Here's how the part is built. I have some questions about the finished solid (model axes, mm). A direction names the side the tool comes from. Give positions to 0.01 mm unless a question says otherwise; leave off trailing zeros. Loops run counter-clockwise (first coordinate to the right, second up) from the corner with the lowest first, then second, coordinate; pieces in that order, holes last. Notation, with made-up numbers: (62, 57.25) - (70, 57.25) arc R27 cw to (70, 75.25) - close; hole circle Ø5 at (56.25, -5). An arc over 180 degrees is marked (long way). Use one line per item in the form item = value.
from build123d import *

# Parameters (mm, degrees)
SKETCH1_R                = 24.193
SKETCH1_R_2              = 20.193
BOSS_EXTRUDE1_DEPTH      = 24
CUT_EXTRUDE1_DEPTH       = 24
BOSS_EXTRUDE2_DEPTH      = 24
SKETCH4_R                = 4
CUT_EXTRUDE2_DEPTH       = 24
SKETCH6_R                = 4
BOSS_EXTRUDE3_DEPTH      = 9.2
BOSS_EXTRUDE3_DEPTH_BACK = 11
SKETCH6_5_R              = 4
CUT_EXTRUDE4_DEPTH       = 4.5


with BuildPart() as part:
    # Sketch1 → Boss-Extrude1 (new body)
    with BuildSketch(Plane.XY):
        Circle(SKETCH1_R)
        Circle(SKETCH1_R_2, mode=Mode.SUBTRACT)
    extrude(amount=BOSS_EXTRUDE1_DEPTH)

    # Sketch2 → Cut-Extrude1 (cut)
    with BuildSketch(Plane.XY.offset(24)):
        Polygon((0, -24.193), (-5.8341998, -24.895299835), (-12.0965, -20.951752594), (0, 0), align=None)
    extrude(amount=-CUT_EXTRUDE1_DEPTH, mode=Mode.SUBTRACT)

    # Sketch3 → Boss-Extrude2 (add)
    with BuildSketch(Plane.XY.offset(24)):
        with BuildLine():
            Line((-15.990029306, -35.482601784), (-12.0965, -20.951752594))
            ThreePointArc((-12.0965, -20.951752594), (-14.346719144, -19.480064138), (-16.419734671, -17.767767512))
            Line((-16.419734671, -17.767767512), (-20.819658437, -34.188506559))
            Line((-20.819658437, -34.188506559), (-15.990029306, -35.482601784))
        make_face()
        with BuildLine():
            ThreePointArc((5.336023592, -23.597205369), (2.684591171, -24.043589982), (0, -24.193))
            Line((0, -24.193), (-3.893529306, -38.72384919))
            Line((-3.893529306, -38.72384919), (0.936099826, -40.017944416))
            Line((0.936099826, -40.017944416), (5.336023592, -23.597205369))
        make_face()
    extrude(amount=-BOSS_EXTRUDE2_DEPTH)

    # Sketch4 → Cut-Extrude2 (cut)
    with BuildSketch(Plane(origin=(-10.877879131, 2.914718929, 0), x_dir=(0, 0, 1), z_dir=(-0.965925826, 0.258819045, 0))):
        with Locations((12, -30.412085563)):
            Circle(SKETCH4_R)
    extrude(amount=-CUT_EXTRUDE2_DEPTH, mode=Mode.SUBTRACT)

    # Sketch6 → Boss-Extrude3 (add, two sides)
    with BuildSketch(Plane(origin=(7.790062397, 29.072908658, 0), x_dir=(0.965925826, -0.258819045, 0), z_dir=(-0.258819045, -0.965925826, 0))) as boss_extrude3_sk:
        Polygon((9.812840635, 15.244290606), (-27.270593421, 0), (26.757277212, 0), align=None)
        Polygon((-34.874772554, 18.498012318), (-27.270593421, 0), (9.812840635, 15.244290606), (26.757277212, 0), (34.96828798, -7.387146438), (48.34481793, 7.481224235), (13.840171432, 38.52379423), align=None)
        with Locations((33.971441151, 6.96105325)):
            Circle(SKETCH6_R, mode=Mode.SUBTRACT)
        with Locations((19.103070478, 20.337583201)):
            Circle(SKETCH6_R, mode=Mode.SUBTRACT)
        Polygon((-37.726339728, 25.434766937), (-34.874772554, 18.498012318), (13.840171432, 38.52379423), (48.34481793, 7.481224235), (53.361016662, 13.056863238), (15.35042048, 47.253608089), align=None)
    extrude(amount=BOSS_EXTRUDE3_DEPTH)
    extrude(boss_extrude3_sk.sketch, amount=-BOSS_EXTRUDE3_DEPTH_BACK)

    # Sketch6_5 → Cut-Extrude4 (cut)
    with BuildSketch(Plane(origin=(7.790062397, 29.072908658, 0), x_dir=(0.965925826, -0.258819045, 0), z_dir=(-0.258819045, -0.965925826, 0))):
        Polygon((-34.874772554, 18.498012318), (-27.270593421, 0), (9.812840635, 15.244290606), (26.757277212, 0), (34.96828798, -7.387146438), (48.34481793, 7.481224235), (13.840171432, 38.52379423), align=None)
        with Locations((33.971441151, 6.96105325)):
            Circle(SKETCH6_5_R, mode=Mode.SUBTRACT)
        with Locations((19.103070478, 20.337583201)):
            Circle(SKETCH6_5_R, mode=Mode.SUBTRACT)
        Polygon((9.812840635, 15.244290606), (-27.270593421, 0), (26.757277212, 0), align=None)
    extrude(amount=-CUT_EXTRUDE4_DEPTH, mode=Mode.SUBTRACT)


solid = part.part
(1) If we section it at B-B (z = 4.5): List the corners of the cut face in (x, y) for me.
Geometry says:
outline = (-22.72, 27.72) - (-6.36, 23.34) arc R24.19 ccw to (-16.42, -17.77) - (-20.82, -34.19) - (-15.99, -35.48) - (-12.1, -20.95) - (-10.1, -17.49) arc R20.19 cw (long way) to (0, -20.19) - (0, -24.19) - (-3.89, -38.72) - (0.94, -40.02) - (5.34, -23.6) arc R24.19 ccw to (17.18, 17.03) - (35.18, 12.21) - (37.56, 21.1) - (-20.34, 36.61) - close; (-19.17, 40.96) - (38.72, 25.44) - (40.41, 31.72) - (-17.49, 47.24) - close; (41.27, 10.58) - (49.52, 8.37) - (51.9, 17.25) - (43.65, 19.46) - close; (44.81, 23.81) - (53.06, 21.6) - (54.74, 27.88) - (46.5, 30.09) - close
(2) If we section it at D-D (z = 36): List the corners of the cut face in (x, y) for me.
Geometry says:
outline = (-6.21, 23.3) - (32.32, 12.98) - (37.55, 32.49) - (-0.98, 42.81) - close; hole (15.23, 27.08) - (23.87, 24.76) - (25.03, 29.11) - (16.39, 31.43) - close
(3) If we section it at A-A (y = 0): List the corners of the cut face in (x, z) for me.
Geometry says:
outline = (-24.19, 0) - (-20.19, 0) - (-20.19, 24) - (-24.19, 24) - close; (20.19, 0) - (24.19, 0) - (24.19, 24) - (20.19, 24) - close
(4) If we section it at C-C (x = 16): List the corners of the cut face in (y, z) for me, plus the area to 3 significant figures.
Geometry says:
outline = (-18.15, 0) - (-12.32, 0) - (-12.32, 24) - (-18.15, 24) - close; (12.32, 0) - (26.87, 0) - (26.87, 36.33) - (31.53, 35.83) - (31.53, 0) - (38.26, 0) - (38.26, 43.23) - (17.35, 45.45) - (17.35, 24) - (12.32, 24) - close
area = 1,020 mm²
(5) For P1, Ø2, axis at x = 49.5, z = 19, coming from the -Y side; P2, Ø5, axis at x = -14.5, z = 9, coming from the -Y side; P3, Ø3, axis at y = -21.5, z = 12.5, coming from the -X side; P4, Ø8, axis at x = 31, y = -3, coming from the -Z side, each with a flat end and sliding along its axis, tell me the tip position at first contact or that it passes through.
Geometry says:
P1 = 8.1
P2 = -35.48
P3 = -17.77
P4 = through
(6) For faces 4 (the flat face through (-17.61, -22.21, 12.17)), 5 (the flat face through (-11.11, -19.24, 12.17)), 6 (the flat face through (0, -22, 12)), which set-ups out of +Z, -Z, +X, -X, +Y, -Y let a thin tool reach every point of the face, with its end or its side?
Geometry says:
face_4 = +Z, -Z, -X
face_5 = +Z, -Z, -Y
face_6 = +Z, -Z
(7) If I drill on probe 1 along X at (y, z) = (0, 12); probe 2 along Z at (x, y) = (-15, 14); probe 3 along Z at (x, y) = (30.5, 32.5), over which ranges is the centre line in solid material (lowest first)?
Geometry says:
probe_1 = -24.19 to -20.19, 20.19 to 24.19
probe_2 = 0 to 24
probe_3 = 0 to 16.84, 23.83 to 42.13
(8) Thinking about a two-plate mould opening in Z: for faces 1 (the flat face through (-2.461, 32.605, 36.497)), 2 (the cylindrical face through (22.002, 20.569, 17.904)), 3 (the flat face through (36.338, 16.594, -3.642)), which applies, pulls with the +Z half, pulls with the -Z half, needs draft (parallel to the pull), parting line crosses it, or undercut?
Geometry says:
face_1 = pulls with the +Z half
face_2 = undercut
face_3 = pulls with the -Z half
